Here's how the part is built. I have some questions about the finished solid (model axes, mm). A direction names the side the tool comes from. Coordinates: 2 decimals unless noted, no trailing zeros. Write each loop counter-clockwise with the first axis right and the second up, starting at its lowest first coordinate (ties: lowest second). Pieces come first, ordered by that corner, then holes. Notation, with made-up numbers: M 14,-19 L 62,-19 A34 cw 62,19 Z; hole C 53.25,21 d10. An arc over 180 degrees is marked long. Use one line per item in the form item = value. Start each with the question number.
1. I want a section at C-C, the plane z = 8.5. List the corners of the cut face in (x, y) for me.
2. Thinking about a two-plate mould opening in X: for faces 1 (the face through (-20, 10, 11)), 2 (the face through (1.32, 4.93, -29.97)), 3 (the face through (-0.08, 5.07, 27.75)), which applies, released by +X, released by -X, zero draft, split by the parting line, or undercut?
3. I want a section at A-A, the plane x = 0. List the corners of the cut face in (y, z) for me, plus the area to 3 significant figures.
4. I want a section at D-D, the plane y = 4.5. Count the separate pieces of the cut face and the enclosed holes in it, plus the area to 3 significant figures.
5. I'm going to push flat-ended pins straight in: pin 1 Ø3 at (x, z) = (18.38, -18.38) entering from +Y; pin 2 Ø3 at (y, z) = (5, 5.5) entering from -X; pin 3 Ø5 at (x, z) = (-7, 11) entering from +Y; pin 4 Ø3 at (y, z) = (2.5, 16.5) entering from -X. Where does each tip first touch, or does it pass through?
6. On a 3-axis mill with a long thin cutter (end or side, diameter ignored), from which of +Z, -Z, +X, -X, +Y, -Y can I reach the whole of each face in a straight line? I mean faces 4 (the face through (15.3, 9, -0.3)), 5 (the face through (19.773, 5.07, -17.319)). Say none if no direction works.
7. I want a section at B-B, the plane z = 0. List the corners of the cut face in (x, y) for me, plus the area to 3 significant figures.
8. Please list where these lines run through material, in increasing order: line 1 along X through (y, z) = (2.25, -13); line 2 along X through (y, z) = (8.25, -17); line 3 along Z through (x, y) = (1, 7.25). Write a range as [from, to].
from build123d import *

# Parameters (mm, degrees)
SKETCH1_R           = 30
BOSS_EXTRUDE1_DEPTH = 10
SKETCH2_R           = 15
CUT_EXTRUDE1_DEPTH  = 44.588989435
SKETCH3_R           = 22.5
CUT_EXTRUDE2_DEPTH  = 1
SKETCH4_R           = 1.75
CUT_EXTRUDE3_DEPTH  = 44.370496884
CIRPATTERN1_COUNT   = 8
SKETCH5_R           = 1.75
CUT_EXTRUDE4_DEPTH  = 44.588989435
CIRPATTERN2_COUNT   = 8


with BuildPart() as part:
    # Sketch1 → Boss-Extrude1 (new body)
    with BuildSketch(Plane(origin=(0, 0, 0), x_dir=(1, 0, 0), z_dir=(0, 1, 0))):
        with Locations(Location((0, 0, 0), (0, 0, 270))):
            Circle(SKETCH1_R)
    extrude(amount=BOSS_EXTRUDE1_DEPTH)

    # Sketch2 → Cut-Extrude1 (cut, through all)
    with BuildSketch(Plane(origin=(0, 10, 0), x_dir=(1, 0, 0), z_dir=(0, 1, 0))):
        with Locations(Location((0, 0, 0), (0, 0, 270))):
            Circle(SKETCH2_R)
    extrude(amount=-CUT_EXTRUDE1_DEPTH, mode=Mode.SUBTRACT)

    # Sketch3 → Cut-Extrude2 (cut)
    with BuildSketch(Plane(origin=(0, 10, 0), x_dir=(1, 0, 0), z_dir=(0, 1, 0))):
        with Locations(Location((0, 0, 0), (0, 0, 270))):
            Circle(SKETCH3_R)
    extrude(amount=-CUT_EXTRUDE2_DEPTH, mode=Mode.SUBTRACT)

    # Sketch4 → Cut-Extrude3 (cut, through all)
    with BuildSketch(Plane(origin=(0, 9, 0), x_dir=(1, 0, 0), z_dir=(0, 1, 0))):
        with Locations(Location((0, 18.5, 0), (0, 0, 270))):
            Circle(SKETCH4_R)
    cut_extrude3 = extrude(amount=-CUT_EXTRUDE3_DEPTH, mode=Mode.SUBTRACT)

    # CirPattern1: Cut-Extrude3 ×8 about axis
    cirpattern1_axis = Axis((0, 0, 0), (0, 1, 0))
    for i in range(1, CIRPATTERN1_COUNT):
        add(cut_extrude3.rotate(cirpattern1_axis, i * 360 / CIRPATTERN1_COUNT), mode=Mode.SUBTRACT)

    # Sketch5 → Cut-Extrude4 (cut, through all)
    with BuildSketch(Plane(origin=(0, 10, 0), x_dir=(1, 0, 0), z_dir=(0, 1, 0))):
        with Locations(Location((0, 26, 0), (0, 0, 270))):
            Circle(SKETCH5_R)
    cut_extrude4 = extrude(amount=-CUT_EXTRUDE4_DEPTH, mode=Mode.SUBTRACT)

    # CirPattern2: Cut-Extrude4 ×8 about axis
    cirpattern2_axis = Axis((0, 0, 0), (0, 1, 0))
    for i in range(1, CIRPATTERN2_COUNT):
        add(cut_extrude4.rotate(cirpattern2_axis, i * 360 / CIRPATTERN2_COUNT), mode=Mode.SUBTRACT)


solid = part.part
Answer list:
q1.outline = M -28.77,0 L -12.36,0 L -12.36,9 L -20.83,9 L -20.83,10 L -28.77,10 Z; M 12.36,0 L 28.77,0 L 28.77,10 L 20.83,10 L 20.83,9 L 12.36,9 Z
q2.face_1 = zero draft
q2.face_2 = split by the parting line
q2.face_3 = undercut
q3.outline = M 0,-30 L 10,-30 L 10,-27.75 L 0,-27.75 Z; M 0,-24.25 L 10,-24.25 L 10,-22.5 L 9,-22.5 L 9,-20.25 L 0,-20.25 Z; M 0,-16.75 L 9,-16.75 L 9,-15 L 0,-15 Z; M 0,15 L 9,15 L 9,16.75 L 0,16.75 Z; M 0,20.25 L 9,20.25 L 9,22.5 L 10,22.5 L 10,24.25 L 0,24.25 Z; M 0,27.75 L 10,27.75 L 10,30 L 0,30 Z
q3.area = 152 mm²
q4.separate_pieces = 1
q4.enclosed_holes = 17
q4.area = 1,970 mm²
q5.pin_1 = through
q5.pin_2 = -29.73
q5.pin_3 = 9
q5.pin_4 = -25.98
q6.face_4 = +Y
q6.face_5 = +Y, -Y
q7.outline = M -30,0 L -27.75,0 L -27.75,10 L -30,10 Z; M -24.25,0 L -20.25,0 L -20.25,9 L -22.5,9 L -22.5,10 L -24.25,10 Z; M -16.75,0 L -15,0 L -15,9 L -16.75,9 Z; M 15,0 L 16.75,0 L 16.75,9 L 15,9 Z; M 20.25,0 L 24.25,0 L 24.25,10 L 22.5,10 L 22.5,9 L 20.25,9 Z; M 27.75,0 L 30,0 L 30,10 L 27.75,10 Z
q7.area = 152 mm²
q8.line_1 = [-27.04, -14.83], [-11.33, -7.48], [7.48, 11.33], [14.83, 27.04]
q8.line_2 = [-24.72, -19.45], [-17.31, -0.9], [0.9, 17.31], [19.45, 24.72]
q8.line_3 = [-29.98, -27.44], [-24.56, -19.94], [-17.06, -14.97], [14.97, 17.06], [19.94, 24.56], [27.44, 29.98]
